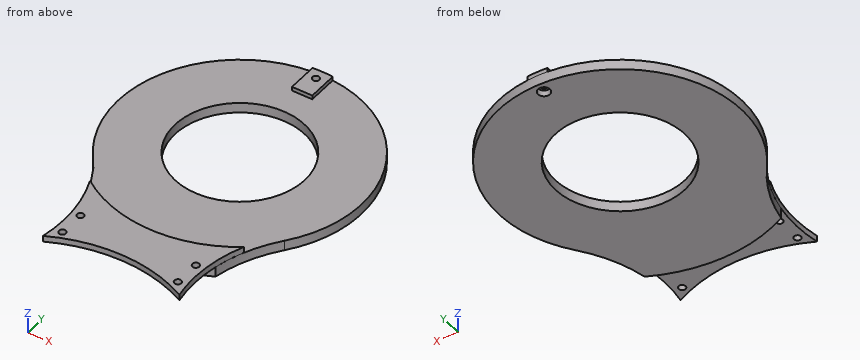
```python
from build123d import *

# Parameters (mm, degrees)
SKETCH_R        = 32
PAD_DEPTH       = 5
PAD001_DEPTH    = 2
SKETCH002_R     = 1.7
POCKET_DEPTH    = 7.001
SKETCH003_R     = 2.95
POCKET001_DEPTH = 3
SKETCH004_R     = 1.7
POCKET002_DEPTH = 7.001
POCKET004_DEPTH = 7.001
SKETCH007_R     = 1.7
PAD002_DEPTH    = 3


with BuildPart() as part:
    # Sketch → Pad (new body)
    with BuildSketch(Plane.XY):
        with BuildLine():
            ThreePointArc((-47.293619, 36.923077), (0, -60), (47.293619, 36.923077))
            ThreePointArc((47.293619, 123.076923), (32.469508, 80), (47.293619, 36.923077))
            ThreePointArc((47.293619, 123.076923), (3.1e-05, 220), (-47.293657, 123.076972))
            ThreePointArc((-47.293619, 36.923077), (-32.469508, 80.000031), (-47.293657, 123.076972))
        make_face()
        Circle(SKETCH_R, mode=Mode.SUBTRACT)
        with Locations((0, 160)):
            Circle(SKETCH_R, mode=Mode.SUBTRACT)
    extrude(amount=PAD_DEPTH)

    # Sketch001 (on Face8 of Pad) → Pad001 (join)
    with BuildSketch(Plane.XY.offset(5)):
        with BuildLine():
            Line((-5, -59.791304), (-5, -45))
            Line((-5, -45), (5, -45))
            Line((5, -45), (5, -59.791304))
            ThreePointArc((-5, -59.791304), (0, -60), (5, -59.791304))
        make_face()
        with BuildLine():
            ThreePointArc((5, 219.791304), (0, 220), (-5, 219.791304))
            Line((-5, 219.791304), (-5, 205))
            Line((-5, 205), (5, 205))
            Line((5, 205), (5, 219.791304))
        make_face()
    extrude(amount=PAD001_DEPTH)

    # Sketch002 (on Face14 of Pad001) → Pocket (cut, through all)
    with BuildSketch(Plane.XY.offset(7)):
        with Locations((0, -55)):
            Circle(SKETCH002_R)
        with Locations((0, 215)):
            Circle(SKETCH002_R)
    extrude(amount=-POCKET_DEPTH, mode=Mode.SUBTRACT)

    # Sketch003 (on Face4 of Pocket) → Pocket001 (cut)
    with BuildSketch(Plane(origin=(0, 0, 0), x_dir=(1, 0, 0), z_dir=(0, 0, -1))):
        with Locations((0, 55)):
            Circle(SKETCH003_R)
        with Locations((0, -215)):
            Circle(SKETCH003_R)
    extrude(amount=-POCKET001_DEPTH, mode=Mode.SUBTRACT)

    # Sketch004 (on Face4 of Pocket001) → Pocket002 (cut, through all)
    with BuildSketch(Plane(origin=(0, 0, 0), x_dir=(1, 0, 0), z_dir=(0, 0, -1))):
        with Locations((28.5, -73.5)):
            Circle(SKETCH004_R)
        with Locations((28.5, -86.5)):
            Circle(SKETCH004_R)
        with Locations((-28.5, -86.5)):
            Circle(SKETCH004_R)
        with Locations((-28.5, -73.5)):
            Circle(SKETCH004_R)
    extrude(amount=-POCKET002_DEPTH, mode=Mode.SUBTRACT)

    # Sketch006 (on Face4 of Pocket002) → Pocket004 (cut, through all)
    with BuildSketch(Plane(origin=(0, 0, 0), x_dir=(1, 0, 0), z_dir=(0, 0, -1))):
        with BuildLine():
            ThreePointArc((65, -122.583426), (0, -85), (-65, -122.583426))
            Line((-65, -122.583426), (-65, 77.416574))
            Line((-65, 77.416574), (65, 77.416574))
            Line((65, 77.416574), (65, -122.583426))
        make_face()
    extrude(amount=-POCKET004_DEPTH, mode=Mode.SUBTRACT)

    # Sketch007 (on Face4 of Pocket004) → Pad002 (join)
    with BuildSketch(Plane.XY.offset(5)):
        with BuildLine():
            ThreePointArc((33.68542, 67.009644), (0, 75), (-33.68542, 67.009644))
            ThreePointArc((-33.68542, 67.009644), (-32.867557, 87.454427), (-37.996513, 107.2623))
            ThreePointArc((-37.996513, 107.2623), (0, 95), (37.996513, 107.2623))
            ThreePointArc((37.996513, 107.2623), (32.867557, 87.454427), (33.68542, 67.009644))
        make_face()
        with Locations((-28.5, 86.5)):
            Circle(SKETCH007_R, mode=Mode.SUBTRACT)
        with Locations((-28.5, 73.5)):
            Circle(SKETCH007_R, mode=Mode.SUBTRACT)
        with Locations((28.5, 73.5)):
            Circle(SKETCH007_R, mode=Mode.SUBTRACT)
        with Locations((28.5, 86.5)):
            Circle(SKETCH007_R, mode=Mode.SUBTRACT)
    extrude(amount=PAD002_DEPTH)


solid = part.part
```
Design review of the part built by this model. Coordinates are the model's own, in mm. Coordinates: 2 decimals unless noted, no trailing zeros. Loops run counter-clockwise (first coordinate to the right, second up) from the corner with the lowest first, then second, coordinate; pieces in that order, holes last. Notation, with made-up numbers: (17, -38.75) - (55, -38.75) arc R14 ccw to (55, -33.75) - close; hole circle Ø11 at (58, -16.75). An arc over 180 degrees is marked (long way). Use CSV: the item, a comma, the result in double quotes. Start each with the question number.
1) Consider section B-B on x = 0. Write out the cut boundary in (y, z), then the cut area to 3 significant figures.
2) Wall thickness on L1, parallel to Y at x = 0, z = 4.5; L2, parallel to X at y = 86.5, z = 6.65; L3, parallel to Z at x = -49, y = 189.5: over which ranges is each line inside the solid? List them lowest first. Write a range as from..to.
3) Consider section A-A on y = 160. Write out the cut boundary in (x, z), then the cut area to 3 significant figures.
4) For pin 1 Ø1.8 at (x, y) = (-0.5, 216.5) entering from -Z; pin 2 Ø5.5 at (x, y) = (0, 215) entering from +Z; pin 3 Ø2 at (x, z) = (2, 6) entering from -Y; pin 4 Ø2 at (x, y) = (28.5, 86.5) entering from -Z, all flat-tipped, find the tip position at first contact; note any pin that passes through.
Geometry says:
1,outline,"(75, 5) - (85, 5) - (85, 0) - (128, 0) - (128, 5) - (95, 5) - (95, 8) - (75, 8) - close; (192, 0) - (212.05, 0) - (212.05, 3) - (213.3, 3) - (213.3, 7) - (205, 7) - (205, 5) - (192, 5) - close; (216.7, 3) - (217.95, 3) - (217.95, 0) - (220, 0) - (220, 7) - (216.7, 7) - close"
1,area,"414 mm^2"
2,L1,"85..128, 192..213.3, 216.7..220"
2,L2,"-32.77..-30.2, -26.8..26.8, 30.2..32.77"
2,L3,"0..5"
3,outline,"(-60, 0) - (-32, 0) - (-32, 5) - (-60, 5) - close; (32, 0) - (60, 0) - (60, 5) - (32, 5) - close"
3,area,"280 mm^2"
4,pin 1,"z = 3"
4,pin 2,"z = 7"
4,pin 3,"y = 74.94"
4,pin 4,"through"
